```python
from build123d import *

# Parameters (mm, degrees)
F2_R     = 3
F3_DEPTH = 20.001
F4_R     = 5
F5_DEPTH = 6


with BuildPart() as f1:
    # F0 (on Front) → F1 (revolve)
    with BuildSketch(Plane.XZ):
        Polygon((11, 20), (11, 0), (20, 0), (20, 12), (40, 12), (40, 20), align=None)
    revolve(axis=Axis((0, 0, 10), (0, 0, 1)))

    # F2 (on face) → F3 (cut, through all)
    with BuildSketch(Plane.XY.offset(20)):
        with Locations((0, 32.5)):
            Circle(F2_R)
        with Locations((-32.5, 0)):
            Circle(F2_R)
        with Locations((0, -32.5)):
            Circle(F2_R)
        with Locations((32.5, 0)):
            Circle(F2_R)
    extrude(amount=-F3_DEPTH, mode=Mode.SUBTRACT)

    # F4 (on face) → F5 (cut)
    with BuildSketch(Plane.XY.offset(20)):
        with Locations((0, 32.5)):
            Circle(F4_R)
        with Locations((-32.5, 0)):
            Circle(F4_R)
        with Locations((0, -32.5)):
            Circle(F4_R)
        with Locations((32.5, 0)):
            Circle(F4_R)
    extrude(amount=-F5_DEPTH, mode=Mode.SUBTRACT)


solid = f1.part
```
Model file for the job. Use its own axes, mm. A direction names the side the tool comes from. Coordinates: 2 decimals unless noted, no trailing zeros. Write each loop counter-clockwise with the first axis right and the second up, starting at its lowest first coordinate (ties: lowest second). Pieces come first, ordered by that corner, then holes. Notation, with made-up numbers: (60, -18) - (88, -18) arc R24 cw to (88, 15) - close; hole circle Ø4 at (68.25, 82.25). An arc over 180 degrees is marked (long way). One line per question, with ' | ' between items. Start each with the question number.
Q1. Cut at B-B, the plane y = -9. List the corners of the cut face in (x, z), then the cut area to 3 significant figures.
Q2. Drill centre lines: line 1 (Y direction, x = 0, z = 17.7); line 2 (Y direction, x = 0, z = 13.45); line 3 (Y direction, x = 0, z = 8.25). Where is each one in solid material? Low to high. Write a range as [from, to].
Q3. Cut at A-A, the plane x = 0. List the corners of the cut face in (y, z).
Q4. Pin check, flat tips, straight feed: pin 1 (6 mm diameter, centred on x = 12, z = 7, fed in from +Y); pin 2 (16 mm diameter, centred on x = -32.5, y = 0, fed in from -Z); pin 3 (4 mm diameter, centred on x = 30.5, z = 12, fed in from -Y). Stop position of each tip, or through.
Q5. Cut at C-C, the plane x = -32.5. List the corners of the cut face in (y, z).
Q6. 3-axis set-ups, long thin cutter, end or side, ignore diameter. For faces 1 (the face through (-0.65, -35.43, 13.01)), 2 (the face through (-1.08, -37.38, 17.04)): which of +Z, -Z, +X, -X, +Y, -Y reach the whole face in a straight line?
Q7. Cut at D-D, the plane y = -1. List the corners of the cut face in (x, z), then the cut area to 3 significant figures.
Q8. Pull direction X, two halves, no side cores. Call faces 3 (the face through (-4.336, -19.524, 6.084)), 4 (the face through (-30, -2, 14)), 5 (the face through (9.4, 18.3, 12)): pulls with the +X half, pulls with the -X half, needs draft (parallel to the pull), parting line crosses it, or undercut.
Answer below:
1) outline: (-38.97, 12) - (-17.86, 12) - (-17.86, 0) - (-6.32, 0) - (-6.32, 20) - (-38.97, 20) - close; (6.32, 0) - (17.86, 0) - (17.86, 12) - (38.97, 12) - (38.97, 20) - (6.32, 20) - close | area: 799 mm^2
2) line 1: [-40, -37.5], [-27.5, -11], [11, 27.5], [37.5, 40] | line 2: [-40, -35.5], [-29.5, -11], [11, 29.5], [35.5, 40] | line 3: [-20, -11], [11, 20]
3) outline: (-40, 12) - (-35.5, 12) - (-35.5, 14) - (-37.5, 14) - (-37.5, 20) - (-40, 20) - close; (-29.5, 12) - (-20, 12) - (-20, 0) - (-11, 0) - (-11, 20) - (-27.5, 20) - (-27.5, 14) - (-29.5, 14) - close; (11, 0) - (20, 0) - (20, 12) - (29.5, 12) - (29.5, 14) - (27.5, 14) - (27.5, 20) - (11, 20) - close; (35.5, 12) - (40, 12) - (40, 20) - (37.5, 20) - (37.5, 14) - (35.5, 14) - close
4) pin 1: y = 17.86 | pin 2: z = 12 | pin 3: y = -28.07
5) outline: (-23.32, 12) - (-3, 12) - (-3, 14) - (-5, 14) - (-5, 20) - (-23.32, 20) - close; (3, 12) - (23.32, 12) - (23.32, 20) - (5, 20) - (5, 14) - (3, 14) - close
6) face 1: +Z, -Z | face 2: +Z
7) outline: (-39.99, 12) - (-35.33, 12) - (-35.33, 14) - (-37.4, 14) - (-37.4, 20) - (-39.99, 20) - close; (-29.67, 12) - (-19.97, 12) - (-19.97, 0) - (-10.95, 0) - (-10.95, 20) - (-27.6, 20) - (-27.6, 14) - (-29.67, 14) - close; (10.95, 0) - (19.97, 0) - (19.97, 12) - (29.67, 12) - (29.67, 14) - (27.6, 14) - (27.6, 20) - (10.95, 20) - close; (35.33, 12) - (39.99, 12) - (39.99, 20) - (37.4, 20) - (37.4, 14) - (35.33, 14) - close | area: 541 mm^2
8) face 3: parting line crosses it | face 4: undercut | face 5: needs draft
